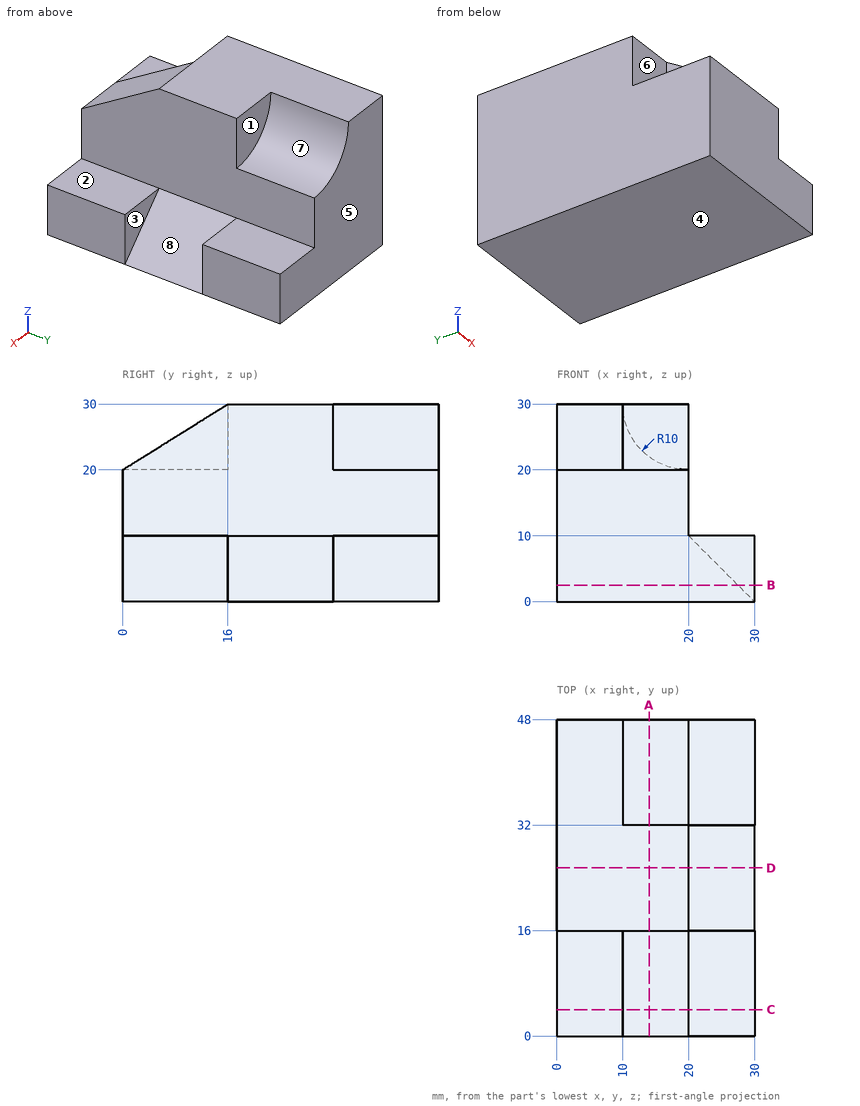
Here's the drawing with two shaded views (mm, measured from the low corner). I have some questions. A direction names the side the tool comes from. Coordinates: 2 decimals unless noted, no trailing zeros. Loops run counter-clockwise (first coordinate to the right, second up) from the corner with the lowest first, then second, coordinate; pieces in that order, holes last. Notation, with made-up numbers: (3, 64.25) -> (21, 64.25) arc R6 ccw to (21, 75.25) -> close; hole circle Ø5 at (4, 83.5). An arc over 180 degrees is marked (long way). Put each result on its own line as item: value. Start each with the question number.
Q1. For the marked faces 1, 2, 3 and 4, which set-ups out of +Z, -Z, +X, -X, +Y, -Y let a thin tool reach every point of the face, with its end or its side?
Q2. I want a section at C-C (y = 4). Write out the boundary of the cut face in (x, z).
Q3. If I drill on line 1 (Y direction, x = 26.75, z = 7.25); line 2 (Z direction, x = 21.5, y = 41); line 3 (X direction, y = 23.5, z = 21), over which ranges is the centre line in solid material (lowest first)? Write a range as [from, to].
Q4. Thinking about a two-plate mould opening in Y: for the marked faces 5, 6, 7 and 8, which applies, pulls with the +Y half, pulls with the -Y half, needs draft (parallel to the pull), parting line crosses it, or undercut?
Q5. I'm going to push flat-ended pins straight in: P1, Ø5, axis at x = 5, y = 8.5, coming from the +Z side; P2, Ø3, axis at x = 25, z = 12.5, coming from the -Y side; P3, Ø5, axis at x = 6, z = 23.5, coming from the -Y side; P4, Ø8, axis at x = 25.5, y = 39.5, coming from the +Z side. Where does each tip first touch, or does it pass through?
Q6. I want a section at B-B (z = 2.5). Write out the boundary of the cut face in (x, y).
Q7. I want a section at D-D (y = 25.5). Write out the boundary of the cut face in (x, z), plus the area to 3 significant figures.
Q8. I want a section at A-A (x = 14). Write out the boundary of the cut face in (y, z), plus the area to 3 significant figures.
Taken from the geometry:
1. face 1: +Z, +X, +Y
1. face 2: +Z, +X, +Y, -Y
1. face 3: +Z, +X
1. face 4: -Z, +X, -X, +Y, -Y
2. outline: (0, 0) -> (30, 0) -> (30, 10) -> (20, 10) -> (20, 22.5) -> (10, 22.5) -> (10, 20) -> (0, 20) -> close
3. line 1: y = [0, 16], [32, 48]
3. line 2: z = [0, 10]
3. line 3: x = [0, 20]
4. face 5: pulls with the +Y half
4. face 6: pulls with the -Y half
4. face 7: needs draft
4. face 8: undercut
5. P1: stops at z = 20
5. P2: passes through
5. P3: stops at y = 16
5. P4: stops at z = 10
6. outline: (0, 0) -> (30, 0) -> (30, 16) -> (27.5, 16) -> (27.5, 32) -> (30, 32) -> (30, 48) -> (0, 48) -> close
7. outline: (0, 0) -> (30, 0) -> (20, 10) -> (20, 30) -> (0, 30) -> close
7. area: 650 mm2
8. outline: (0, 0) -> (48, 0) -> (48, 22) -> (32, 22) -> (32, 30) -> (16, 30) -> (0, 20) -> close
8. area: 1,230 mm2
